Could you check a few things on this model? Use its own coordinates, in mm. Face numbers are marked on the shaded views. Coordinates: 2 decimals unless noted, no trailing zeros. Write each loop counter-clockwise with the first axis right and the second up, starting at its lowest first coordinate (ties: lowest second). Pieces come first, ordered by that corner, then holes.
Item 1: I want a section at A-A on y = 21.2. Please give me the cut outline in (x, z).
Item 2: Thinking about a two-plate mould opening in X: for the marked faces 1, 2 and 3, which applies, +X half, -X half, draft (parallel to the pull), parting line (faces both ways), or undercut?
Item 3: I want a section at C-C on y = 7. Please give me the cut outline in (x, z), then the cut area to 3 significant figures.
Item 4: I want a section at B-B on y = 27. Please give me the cut outline in (x, z).
Item 5: If I drill on probe 1 along Y at (x, z) = (0, 4); probe 2 along X at (y, z) = (3.25, 0); probe 3 along Z at (x, y) = (2, 4.5), over which ranges is the centre line in solid material (lowest first)?
Item 6: For P1, Ø6, axis at x = 4.5, z = 1.5, coming from the +Y side; P2, Ø10, axis at x = -1.5, z = 6, coming from the -Y side; P3, Ø5, axis at y = 14, z = 1, coming from the +X side; P4, Ø6, axis at y = 15.5, z = 2, coming from the -X side, each with a flat end and sliding along its axis, tell me the tip position at first contact or that it passes through.
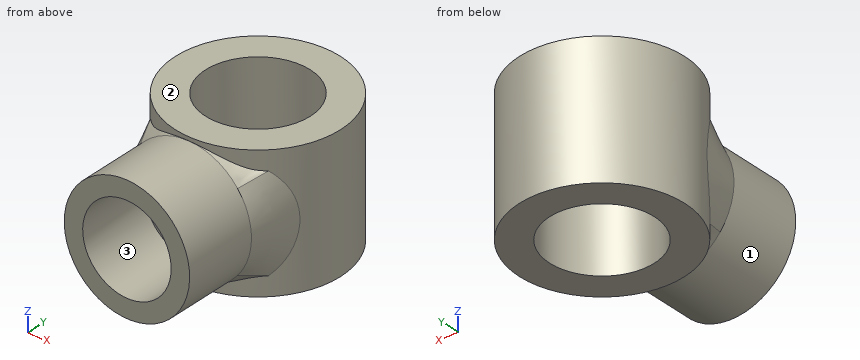
from build123d import *

# Parameters (mm, degrees)
SKETCH1_R                = 8.5
SKETCH1_R_2              = 6
BOSS_EXTRUDE1_DEPTH      = 10
BOSS_EXTRUDE2_DEPTH      = 9
BOSS_EXTRUDE2_DEPTH_BACK = 9
SKETCH3_R                = 11.2
SKETCH8_R                = 7.1
CUT_EXTRUDE1_DEPTH       = 18


with BuildPart() as part:
    # Sketch1 → Boss-Extrude1 (new body)
    with BuildSketch(Plane(origin=(0, 0, 0), x_dir=(1, 0, 0), z_dir=(0, 1, 0))):
        with Locations(Location((0, 0, 0), (0, 0, 270))):
            Circle(SKETCH1_R)
        with Locations(Location((0, 0, 0), (0, 0, 270))):
            Circle(SKETCH1_R_2, mode=Mode.SUBTRACT)
    extrude(amount=BOSS_EXTRUDE1_DEPTH)



with BuildPart() as body_2:
    # Sketch3 → Boss-Extrude2 (new, two sides: drawn at the far end of the back side and taken through both)
    with BuildSketch(Plane.XY.offset(-BOSS_EXTRUDE2_DEPTH_BACK)):
        with Locations((0, 21.2)):
            Circle(SKETCH3_R)
    extrude(amount=BOSS_EXTRUDE2_DEPTH + BOSS_EXTRUDE2_DEPTH_BACK)


with BuildPart() as part_1:
    add(part.part)

    add(body_2.part)  # Loft1 merges body 2
    # Sketch7 → Loft1 section 0
    with BuildSketch(Plane(origin=(0, 21.2, 0), x_dir=(1, 0, 0), z_dir=(0, 1, 0))):
        with BuildLine():
            Line((-11.2, -9), (11.2, -9))
            Line((11.2, -9), (11.2, 9))
            Line((11.2, 9), (-11.2, 9))
            Line((-11.2, 9), (-11.2, -9))
        make_face()
    # Sketch6 for Loft1 → Loft1 section 1
    with BuildSketch(Plane(origin=(0, 10, 0), x_dir=(1, 0, 0), z_dir=(0, 1, 0))):
        with BuildLine():
            # circular arc as an exact rational Bezier (weights 1, cos(half-angle), 1)
            Bezier((-6.625825946, -5.324324421), (0, -13.569796708), (6.625825946, -5.324324421), weights=[1, 0.626391108, 1])
            Bezier((6.625825946, -5.324324421), (10.904300926, 0), (6.625825946, 5.324324421), weights=[1, 0.779508935, 1])
            Bezier((6.625825946, 5.324324421), (0, 13.569796708), (-6.625825946, 5.324324421), weights=[1, 0.626391108, 1])
            Bezier((-6.625825946, 5.324324421), (-10.904300926, 0), (-6.625825946, -5.324324421), weights=[1, 0.779508935, 1])
        make_face()
    loft()

    # Sketch8 → Cut-Extrude1 (cut)
    with BuildSketch(Plane.XY.offset(9)):
        with Locations((0, 21.2)):
            Circle(SKETCH8_R)
    extrude(amount=-CUT_EXTRUDE1_DEPTH, mode=Mode.SUBTRACT)


solid = part_1.part
Response values:
1. outline: (-11.2, -9) - (-7.1, -9) - (-7.1, 9) - (-11.2, 9) - close; (7.1, -9) - (11.2, -9) - (11.2, 9) - (7.1, 9) - close
2. face 1: parting line
2. face 2: draft
2. face 3: undercut
3. outline: circle Ø17 at (0, 0); hole circle Ø12 at (0, 0)
3. area: 114 mm2
4. outline: (-9.58, -9) - (-4.1, -9) - (-4.1, 9) - (-9.58, 9) - close; (4.1, -9) - (9.58, -9) - (9.58, 9) - (4.1, 9) - close
5. probe 1: y = 10 to 14.1, 28.3 to 32.4
5. probe 2: x = -8.5 to -6, 6 to 8.5
5. probe 3: z = -8.26 to -5.66, 5.66 to 8.26
6. P1: stops at y = 32.3
6. P2: stops at y = 0
6. P3: stops at x = 10.17
6. P4: stops at x = -10.87
